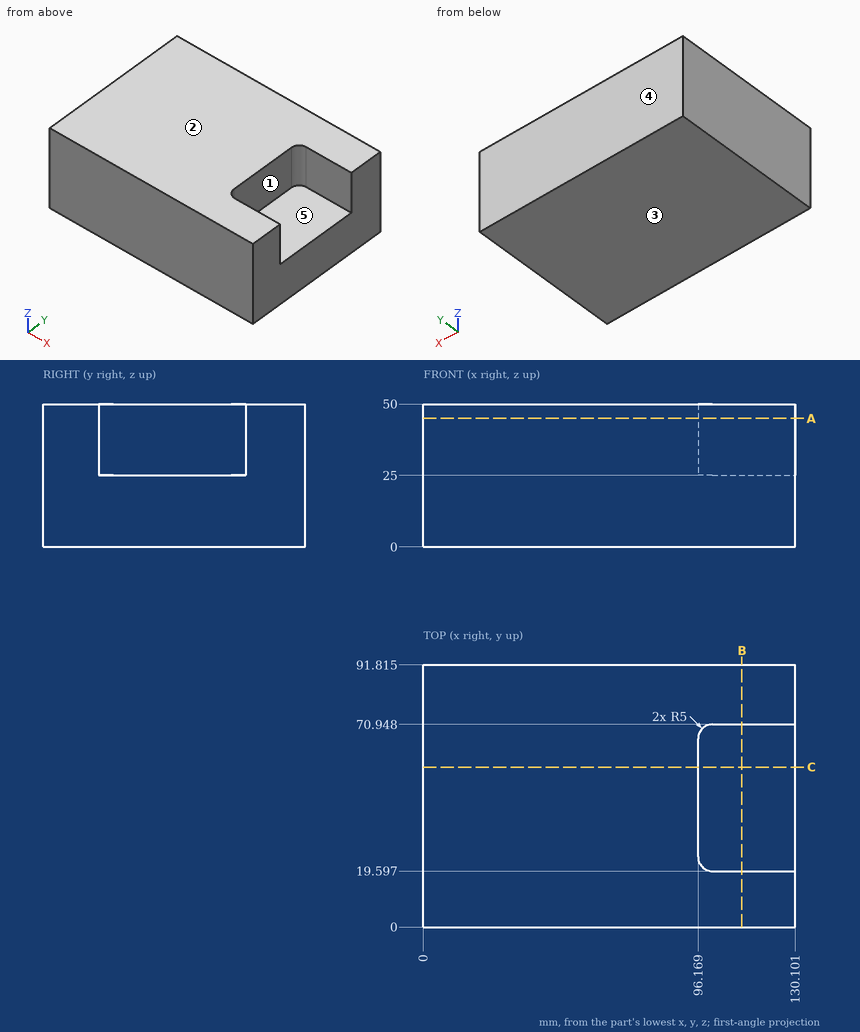
Job drawing, mm, ordinate dimensions from the low corner. One solid piece. A direction names the side the tool comes from. Give positions to 0.01 mm unless a question says otherwise; leave off trailing zeros. Order: outer loops, then holes, each group sorted by start corner. A loop starts at its lowest first (then second) coordinate and runs counter-clockwise, first axis right, second up. Notation, with made-up numbers: (7.25, -24) -> (14.25, -24) arc R11 ccw to (14.25, -8) -> close; hole circle Ø5 at (29.25, -33). An arc over 180 degrees is marked (long way). Return JSON: item names as keys, results as strings.
Q1. Flat gauge pins, fed straight in: pin 1 (10 mm diameter, centred on x = 121, y = 49.5, fed in from +Z); pin 2 (7.5 mm diameter, centred on y = 36.5, z = 33, fed in from +X); pin 3 (8 mm diameter, centred on y = 82, z = 22.5, fed in from -X). Where does each tip first touch, or does it go through?
Working result:
{"pin 1": "z = 25", "pin 2": "x = 96.17", "pin 3": "x = 0"}
Q2. Mould opens along Y. For the marked faces 3, 4 and 5 say: pulls with the +Y half, pulls with the -Y half, needs draft (parallel to the pull), parting line crosses it, or undercut.
Working result:
{"face 3": "needs draft", "face 4": "pulls with the +Y half", "face 5": "undercut"}
Q3. Which spindle directions (+Z, -Z, +X, -X, +Y, -Y) get a long thin tool onto all of the face, cutting with end or side? Do the marked faces 1 and 2. Say none if no direction does.
Working result:
{"face 1": "+Z, +X", "face 2": "+Z, +X, -X, +Y, -Y"}
Q4. Saw through at C-C (y = 56). Write the cut outline in (x, z), then the cut area to 3 significant figures.
Working result:
{"outline": "(0, 0) -> (130.1, 0) -> (130.1, 25) -> (96.17, 25) -> (96.17, 50) -> (0, 50) -> close", "area": "5,660 mm²"}
Q5. Drill centre lines: line 1 (Y direction, x = 111, z = 31) (1 decimal); line 2 (X direction, y = 47.5, z = 35); line 3 (Z direction, x = 104, y = 51). Where is each one in solid material? Low to high.
Working result:
{"line 1": "0 to 19.6, 70.9 to 91.8", "line 2": "0 to 96.17", "line 3": "0 to 25"}
Q6. Saw through at A-A (z = 45). Write the cut outline in (x, y) (1 decimal).
Working result:
{"outline": "(0, 0) -> (130.1, 0) -> (130.1, 19.6) -> (101.2, 19.6) arc R5 cw to (96.2, 24.6) -> (96.2, 65.9) arc R5 cw to (101.2, 70.9) -> (130.1, 70.9) -> (130.1, 91.8) -> (0, 91.8) -> close"}
Q7. Saw through at B-B (x = 111.5). Write the cut outline in (y, z) (1 decimal).
Working result:
{"outline": "(0, 0) -> (91.8, 0) -> (91.8, 50) -> (70.9, 50) -> (70.9, 25) -> (19.6, 25) -> (19.6, 50) -> (0, 50) -> close"}
